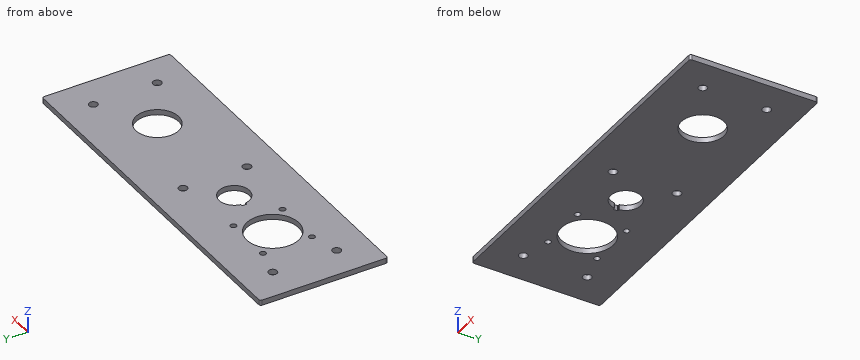
from build123d import *

# Parameters (mm, degrees)
SKETCH1_R             = 12.7
SKETCH1_R_2           = 15.4813
SKETCH1_R_3           = 2.5527
EXTRUDE1_DEPTH        = 3.175
F_6_32_TAPPED_HOLE1_D = 3.5052


with BuildPart() as part:
    # Sketch1 → Extrude1 (new body)
    with BuildSketch(Plane.XY):
        with BuildLine():
            Line((1.27, 38.1), (214.63, 38.1))
            ThreePointArc((214.63, 38.1), (215.528025612, 37.728025612), (215.9, 36.83))
            Line((215.9, 36.83), (215.9, -36.83))
            ThreePointArc((215.9, -36.83), (215.528025612, -37.728025612), (214.63, -38.1))
            Line((214.63, -38.1), (1.27, -38.1))
            ThreePointArc((1.27, -38.1), (0.371974388, -37.728025612), (0, -36.83))
            Line((0, -36.83), (0, 36.83))
            ThreePointArc((0, 36.83), (0.371974388, 37.728025612), (1.27, 38.1))
        make_face()
        with Locations((165.1, 0)):
            Circle(SKETCH1_R, mode=Mode.SUBTRACT)
        with Locations((50.8, 0)):
            Circle(SKETCH1_R_2, mode=Mode.SUBTRACT)
        with Locations((19.05, 19.05)):
            Circle(SKETCH1_R_3, mode=Mode.SUBTRACT)
        with Locations((196.85, 19.05)):
            Circle(SKETCH1_R_3, mode=Mode.SUBTRACT)
        with Locations(Location((196.85, -19.05, 0), (0, 0, 180))):
            Circle(SKETCH1_R_3, mode=Mode.SUBTRACT)
        with Locations(Location((19.05, -19.05, 0), (0, 0, 180))):
            Circle(SKETCH1_R_3, mode=Mode.SUBTRACT)
        with Locations((107.95, 19.05)):
            Circle(SKETCH1_R_3, mode=Mode.SUBTRACT)
        with Locations((107.95, -19.05)):
            Circle(SKETCH1_R_3, mode=Mode.SUBTRACT)
        with BuildLine():
            Line((79.790097811, 1.397), (79.0575, 1.397))
            ThreePointArc((79.0575, 1.397), (78.877894878, 1.322605122), (78.8035, 1.143))
            Line((78.8035, 1.143), (78.8035, -1.143))
            ThreePointArc((78.8035, -1.143), (78.877894878, -1.322605122), (79.0575, -1.397))
            Line((79.0575, -1.397), (79.790097811, -1.397))
            ThreePointArc((79.790097811, -1.397), (79.952903046, -1.456037297), (80.040026541, -1.605705075))
            ThreePointArc((80.040026541, -1.605705075), (97.9043, 0), (80.040026541, 1.605705075))
            ThreePointArc((80.040026541, 1.605705075), (79.952903046, 1.456037297), (79.790097811, 1.397))
        make_face(mode=Mode.SUBTRACT)
    extrude(amount=-EXTRUDE1_DEPTH)

    # #6-32 Tapped Hole1 (through all)
    with Locations(Plane.XY):
        with Locations((36.195, 14.605), (65.405, 14.605), (65.405, -14.605), (36.195, -14.605)):
            Hole(F_6_32_TAPPED_HOLE1_D / 2)


solid = part.part
Could you check a few things on this model? Use its own coordinates, in mm. Give positions to 0.01 mm unless a question says otherwise; leave off trailing zeros. Order: outer loops, then holes, each group sorted by start corner. A loop starts at its lowest first (then second) coordinate and runs counter-clockwise, first axis right, second up. Notation, with made-up numbers: (13, -10) -> (58, -10) arc R22 cw to (58, 20) -> close; hole circle Ø11 at (-15.75, 57.25). An arc over 180 degrees is marked (long way). Return JSON: item names as keys, results as strings.
1. Imagine slicing it at D-D on x = 165.1. List the corners of the cut face in (y, z) for me (3 decimals), then the cut area to 3 significant figures.
Answer list:
{"outline": "(-38.1, -3.175) -> (-12.7, -3.175) -> (-12.7, 0) -> (-38.1, 0) -> close; (12.7, -3.175) -> (38.1, -3.175) -> (38.1, 0) -> (12.7, 0) -> close", "area": "161 mm2"}
2. Imagine slicing it at C-C on z = -1.15. Give the number of separate pieces and of enclosed holes in the cut face, then the cut area to 3 significant figures.
Answer list:
{"separate pieces": "1", "enclosed holes": "13", "area": "14,800 mm2"}
3. I need wall thicknesses on line 1 (Y direction, x = 107.95, z = -1.85); line 2 (X direction, y = -8, z = -0.5); line 3 (X direction, y = 14, z = -2.85). Which ranges of each line are inside material? Lowest first, please. Write a range as from..to.
Answer list:
{"line 1": "y = -38.1..-21.6, -16.5..16.5, 21.6..38.1", "line 2": "x = 0..37.55, 64.05..84.77, 93.03..155.24, 174.96..215.9", "line 3": "x = 0..34.55, 37.84..44.19, 57.41..63.76, 67.05..215.9"}
4. Imagine slicing it at A-A on x = 196.85. List the corners of the cut face in (y, z) for me (3 decimals), then the cut area to 3 significant figures.
Answer list:
{"outline": "(-38.1, -3.175) -> (-21.603, -3.175) -> (-21.603, 0) -> (-38.1, 0) -> close; (-16.497, -3.175) -> (16.497, -3.175) -> (16.497, 0) -> (-16.497, 0) -> close; (21.603, -3.175) -> (38.1, -3.175) -> (38.1, 0) -> (21.603, 0) -> close", "area": "210 mm2"}
5. Imagine slicing it at B-B on y = 19.05. List the corners of the cut face in (x, z) for me (3 decimals), then the cut area to 3 significant figures.
Answer list:
{"outline": "(0, -3.175) -> (16.497, -3.175) -> (16.497, 0) -> (0, 0) -> close; (21.603, -3.175) -> (105.397, -3.175) -> (105.397, 0) -> (21.603, 0) -> close; (110.503, -3.175) -> (194.297, -3.175) -> (194.297, 0) -> (110.503, 0) -> close; (199.403, -3.175) -> (215.9, -3.175) -> (215.9, 0) -> (199.403, 0) -> close", "area": "637 mm2"}
